Could you check a few things on this model? Use its own coordinates, in mm. A direction names the side the tool comes from. Round coordinates to 2 decimals unless told otherwise and drop trailing zeros. Loops run counter-clockwise (first coordinate to the right, second up) from the corner with the lowest first, then second, coordinate; pieces in that order, holes last. Notation, with made-up numbers: (18.5, -34) - (58.5, -34) arc R21 cw to (58.5, -28) - close; hole circle Ø4 at (85, -34.75). An arc over 180 degrees is marked (long way). Use one line per item in the form item = value.
```python
from build123d import *

# Parameters (mm, degrees)
SKETCH_1_R      = 6
EXTRUDE_1_DEPTH = 55
SKETCH_2_R      = 5.25
EXTRUDE_2_DEPTH = 5.5
EXTRUDE_START   = -30
SKETCH_3_R      = 9.5
EXTRUDE_3_DEPTH = 3


with BuildPart() as part:
    # Эскиз1 → Бобышка-Вытянуть1 (new body)
    with BuildSketch(Plane.XY):
        Circle(SKETCH_1_R)
    extrude(amount=EXTRUDE_1_DEPTH)

    # Эскиз2 → Бобышка-Вытянуть2 (add)
    with BuildSketch(Plane.XY.offset(55)):
        Circle(SKETCH_2_R)
    extrude(amount=EXTRUDE_2_DEPTH)

    # Эскиз3 → Бобышка-Вытянуть3 (add)
    with BuildSketch(Plane(origin=(0, 0, 0), x_dir=(-1, 0, 0), z_dir=(0, 0, -1)).offset(EXTRUDE_START)):
        Circle(SKETCH_3_R)
    extrude(amount=EXTRUDE_3_DEPTH)


solid = part.part
```
1. For P1, Ø4, axis at x = -3, y = -5.5, coming from the -Z side; P2, Ø6, axis at y = 1, z = 11, coming from the -X side; P3, Ø3, axis at y = 5, z = 41.5, coming from the +X side; P4, Ø6, axis at x = 6.5, y = 6.5, coming from the +Z side, each with a flat end and sliding along its axis, tell me the tip position at first contact or that it passes through.
Solution:
P1 = 0
P2 = -6
P3 = 4.87
P4 = 30
2. Please list where these lines run through material, in increasing order: line 1 along Z through (x, y) = (-5.25, 7); line 2 along X through (y, z) = (3, 44); line 3 along Y through (x, z) = (1.5, 47.5).
Solution:
line_1 = 27 to 30
line_2 = -5.2 to 5.2
line_3 = -5.81 to 5.81
3. If we section it at A-A, the plane y = 0: Write out the boundary of the cut face in (x, z), plus the area to 3 significant figures.
Solution:
outline = (-9.5, 27) - (-6, 27) - (-6, 0) - (6, 0) - (6, 27) - (9.5, 27) - (9.5, 30) - (6, 30) - (6, 55) - (5.25, 55) - (5.25, 60.5) - (-5.25, 60.5) - (-5.25, 55) - (-6, 55) - (-6, 30) - (-9.5, 30) - close
area = 739 mm^2
4. On a 3-axis mill with a long thin cutter (end or side, diameter ignored), from which of +Z, -Z, +X, -X, +Y, -Y can I reach the whole of each face in a straight line? I mean faces 1 (the face through (0.1, -6.2, 27)), 2 (the face through (0, 0, 60.5)), 3 (the face through (-6, 0, 42)). Say none if no direction works.
Solution:
face_1 = -Z
face_2 = +Z, +X, -X, +Y, -Y
face_3 = +Z
5. If we section it at D-D, the plane y = -6.75: Write out the boundary of the cut face in (x, z).
Solution:
outline = (-6.68, 27) - (6.68, 27) - (6.68, 30) - (-6.68, 30) - close
6. If we section it at C-C, the plane z = 23: Write out the boundary of the cut face in (x, y), plus the area to 3 significant figures.
Solution:
outline = circle Ø12 at (0, 0)
area = 113 mm^2
